Autodesk Fusion 360 part; units mm, degrees
sketch "Sketch1" plane through (0, 0, 0) normal (0, 0, 1) x (1, 0, 0)
  line L0 (0, 0) -> (25.8, 0)
  line L1 (25.8, 0) -> (25.8, -25.8)
  line L2 (0, 0) -> (25.8, 0)
  line L3 (25.8, 0) -> (25.8, -25.8)
  line L4 (25.8, -25.8) -> (0, -25.8)
  line L5 (0, -25.8) -> (0, 0)
  line L6 (25.8, -30.55) -> (-4.75, -30.55)
  line L7 (-4.75, -30.55) -> (-4.75, 4.75)
  line L8 (-4.75, 4.75) -> (25.8, 4.75)
  line L9 (25.8, 0) -> (25.8, 4.75)
  line L10 (25.8, 4.75) -> (25.8, -30.55)
  line L11 (25.8, -12.9) -> (25.8, -62.331)
  line L12 (25.8, -62.331) -> (25.8, -77.331)
  line L13 (25.8, -62.331) -> (25.8, -47.331)
  line L14 (25.8, -47.331) -> (15.8, -47.331)
  line L15 (15.8, -47.331) -> (15.8, -30.55)
  line L16 (15.8, -47.331) -> (15.8, -77.331)
  line L17 (25.8, -77.331) -> (15.8, -77.331)
  dimension "d1" = 25.8
  dimension "d2" = 25.8
  dimension "d4" = 49.431
  dimension "d5" = 15
  dimension "d6" = 15
  dimension "d7" = 10
extrude "Extrude1" add sketch "Sketch1" along normal blind 76.4 contours L0 L2 L4 L5 L6 L7 L8 L9 L10 L11
ref_plane "WorkPlane1" through (10.525, -12.9, 38.2) normal (0, 0, 1) x (1, 0, 0)
extrude "Extrude2" add sketch "Sketch1" along normal mid plane 50 from surface at 38.2 contours L6 L11 L14 L15 | L11 L12 L13 L14 L16 L17
sketch "Sketch2" plane through (15.8, 0, 0) normal (-1, 0, 0) x (0, 0, 1)
  line L0 (13.2, -77.331) -> (63.2, -77.331)
  line L1 (63.2, -77.331) -> (63.2, -30.55)
  line L2 (63.2, -30.55) -> (13.2, -30.55)
  line L3 (13.2, -30.55) -> (13.2, -77.331)
  line L4 (0, -47.331) -> (0, -77.331)
  line L5 (0, -62.331) -> (0, -77.331)
  line L6 (0, -62.331) -> (0, -47.331)
  line L7 (0, -77.331) -> (0, -62.331)
  line L8 (13.2, -62.331) -> (63.2, -62.331) construction
  circle A0 centre (38.2, -62.331) radius 5
  line L9 (63.2, -62.331) -> (60.2, -62.331)
  circle A1 centre (57.65, -62.331) radius 2.55
  line L10 (38.2, -62.331) -> (38.2, -60) construction
  circle A2 centre (18.75, -62.331) radius 2.55
  dimension "d13" = 10
  dimension "d14" = 3
  dimension "d15" = 5.1
extrude "Extrude3" cut sketch "Sketch2" against normal blind 61 contours A1 | A0 | A2
fillet "Fillet1" radius 10 2 edges at (-4.75, -30.55, 38.2) (-4.75, 4.75, 38.2)
fillet "Fillet2" radius 7 2 edges at (20.8, -30.55, 63.2) (20.8, -30.55, 13.2)
fillet "Fillet3" radius 10.5 1 edges at (15.8, -30.55, 38.2)
sketch "Sketch3" plane through (-4.75, 0, 0) normal (-1, 0, 0) x (0, 0, 1)
  line L0 (76.4, -5.25) -> (0, -5.25)
  line L1 (0, -5.25) -> (0, -20.55)
  line L2 (0, -20.55) -> (76.4, -20.55)
  line L3 (76.4, -20.55) -> (76.4, -5.25)
  line L4 (0, -12.9) -> (76.4, -12.9) construction
  circle A0 centre (38.2, -12.9) radius 2.1
  line L5 (38.2, -12.9) -> (58.2, -12.9) construction
  circle A1 centre (58.2, -12.9) radius 2.1
  line L6 (38.2, -12.9) -> (18.2, -12.9) construction
  circle A2 centre (18.2, -12.9) radius 2.1
  dimension "d24" = 4.2
  dimension "d25" = 20
  dimension "d26" = 4.2
  dimension "d27" = 20
  dimension "d28" = 4.2
extrude "Extrude4" cut sketch "Sketch3" against normal blind 40 contours A0 | A1 | A2
sketch "Sketch4" plane through (0, 4.75, 0) normal (0, 1, 0) x (-1, 0, 0)
  line L0 (-5.25, 0) -> (-5.25, 76.4)
  line L1 (-5.25, 76.4) -> (-25.8, 76.4)
  line L2 (-25.8, 76.4) -> (-25.8, 0)
  line L3 (-25.8, 0) -> (-5.25, 0)
  line L4 (4.75, 36.1) -> (4.75, 40.3)
  line L5 (4.75, 16.1) -> (4.75, 20.3)
  line L6 (4.75, 56.1) -> (4.75, 60.3)
  line L7 (4.75, 18.2) -> (-25.8, 18.2) construction
  line L8 (4.75, 38.2) -> (-25.8, 38.2) construction
  line L9 (4.75, 58.2) -> (-25.8, 58.2) construction
  line L10 (-25.8, 18.2) -> (-5.25, 18.2) construction
  line L11 (-5.25, 38.2) -> (-25.8, 38.2)
  line L12 (-25.8, 58.2) -> (-5.25, 58.2)
  circle A0 centre (-15.525, 18.2) radius 2.1
  circle A1 centre (-15.525, 38.2) radius 2.1
  circle A2 centre (-15.525, 58.2) radius 2.1
  point P0 (4.75, 18.2)
  dimension "d31" = 4.2
  dimension "d32" = 4.2
  dimension "d33" = 4.2
extrude "Extrude5" cut sketch "Sketch4" against normal blind 15 contours L11 A1 | L11 A1 | L12 A2 | L12 A2 | A0
Design review of the part built by this model. Coordinates are the model's own, in mm. A direction names the side the tool comes from. Coordinates: 2 decimals unless noted, no trailing zeros. Loops run counter-clockwise (first coordinate to the right, second up) from the corner with the lowest first, then second, coordinate; pieces in that order, holes last. Notation, with made-up numbers: (40.5, 25) -> (73.5, 25) arc R21 cw to (73.5, 60) -> close; hole circle Ø2 at (1.25, 42.5). An arc over 180 degrees is marked (long way). Use a Markdown table: item, result. Add a question column.
Item 1: We need section B-B, the plane x = 21. Write out the cut boundary in (y, z).
Item 2: Wall thickness on L1, parallel to Y at x = 19.5, z = 38.5; L2, parallel to Y at x = 22, z = 29; L3, parallel to Y at x = 18.5, z = 57.65: over which ranges is each line inside the solid? List them lowest first. Write a range as from..to.
Item 3: We need section D-D, the plane x = 2.5. Write out the cut boundary in (y, z).
Item 4: We need section A-A, the plane z = 38.2. Write out the cut boundary in (x, y) (3 decimals), and give its area (3 significant figures).
Item 5: Machinability: for faces 1 (the flat face through (25.8, 2, 38)), 2 (the cylindrical face through (20.73, -61.565, 60.082)), 3 (the cylindrical face through (15.98, 2.41, 36.15)), 4 (the flat face through (15.8, -55, 38)), 5 (the flat face through (20, -57, 63.2)), which of the approach directions +Z, -Z, +X, -X, +Y, -Y give a long, thin tool a straight path to every point of the face, cutting with its end or side? Answer none if there is none.
Item 6: Clearance check with flat-ended pins moving along their axes: P1, Ø8.5, axis at x = 22.5, y = -55, coming from the +Z side; P2, Ø6, axis at x = 16.5, y = -68.5, coming from the -Z side; P3, Ø2.5, axis at x = 15.525, z = 38.2, coming from the +Y side; P4, Ø2.5, axis at y = -12.9, z = 58.2, coming from the +X side. State where each tip first meets the part, or that it passes through.
Item 7: We need section C-C, the plane y = -12.9. Write out the cut boundary in (x, z).
Item 8: The part is to be moulded in two halves that separate along Z. For faces 6 (the cylindrical face through (-2.41, -12.81, 56.1)), 7 (the flat face through (21, -77.331, 38)), 8 (the flat face through (-1, -14, 0)), say which applies: +Z half, -Z half, draft (parallel to the pull), parting line (faces both ways), or undercut.
Numbers:
| question | item | result |
|---|---|---|
| 1 | outline | (-77.33, 13.2) -> (-37.55, 13.2) arc R7 cw to (-30.55, 6.2) -> (-30.55, 0) -> (-25.8, 0) -> (-25.8, 76.4) -> (-30.55, 76.4) -> (-30.55, 70.2) arc R7 cw to (-37.55, 63.2) -> (-77.33, 63.2) -> close; (0, 0) -> (4.75, 0) -> (4.75, 76.4) -> (0, 76.4) -> close; hole circle Ø10 at (-62.33, 38.2); hole circle Ø5.1 at (-62.33, 18.75); hole circle Ø5.1 at (-62.33, 57.65) |
| 2 | L1 | y = -77.33..-67.32, -57.34..-25.8, 0..4.75 |
| 2 | L2 | y = -77.33..-25.8, 0..4.75 |
| 2 | L3 | y = -77.33..-64.88, -59.78..-25.8, 0..4.75 |
| 3 | outline | (-30.16, 0) -> (-25.8, 0) -> (-25.8, 76.4) -> (-30.16, 76.4) -> close; (0, 0) -> (4.36, 0) -> (4.36, 76.4) -> (0, 76.4) -> close |
| 4 | outline | (-4.75, -20.55) arc R10 ccw to (5.25, -30.55) -> (5.3, -30.55) arc R10.5 cw to (15.8, -41.05) -> (15.8, -57.331) -> (25.8, -57.331) -> (25.8, -25.8) -> (0, -25.8) -> (0, -15) -> (-4.75, -15) -> close; (-4.75, -10.8) -> (0, -10.8) -> (0, 0) -> (13.425, 0) -> (13.425, 4.75) -> (5.25, 4.75) arc R10 ccw to (-4.75, -5.25) -> close; (15.8, -77.331) -> (25.8, -77.331) -> (25.8, -67.331) -> (15.8, -67.331) -> close; (17.625, 0) -> (25.8, 0) -> (25.8, 4.75) -> (17.625, 4.75) -> close |
| 4 | area | 721 mm^2 |
| 5 | face 1 | +Z, -Z, +X, +Y, -Y |
| 5 | face 2 | +X, -X |
| 5 | face 3 | +Y |
| 5 | face 4 | +Z, -Z, -X, -Y |
| 5 | face 5 | +Z, +X, -X, -Y |
| 6 | P1 | stops at z = 63.2 |
| 6 | P2 | stops at z = 13.2 |
| 6 | P3 | stops at y = -25.8 |
| 6 | P4 | passes through |
| 7 | outline | (-4.75, 0) -> (0, 0) -> (0, 16.1) -> (-4.75, 16.1) -> close; (-4.75, 20.3) -> (0, 20.3) -> (0, 36.1) -> (-4.75, 36.1) -> close; (-4.75, 40.3) -> (0, 40.3) -> (0, 56.1) -> (-4.75, 56.1) -> close; (-4.75, 60.3) -> (0, 60.3) -> (0, 76.4) -> (-4.75, 76.4) -> close |
| 8 | face 6 | undercut |
| 8 | face 7 | draft |
| 8 | face 8 | -Z half |
